Build history of the part. All positions in model axes, mm. Face numbers are marked on the shaded views. A direction names the side the tool comes from. Coordinates: 2 decimals unless noted, no trailing zeros. Loops run counter-clockwise (first coordinate to the right, second up) from the corner with the lowest first, then second, coordinate; pieces in that order, holes last. Notation, with made-up numbers: (7.5, -9.75) - (46.5, -9.75) arc R32 cw to (46.5, 21.25) - close; hole circle Ø8 at (34, -18.5). An arc over 180 degrees is marked (long way). One line per item, written item: value.
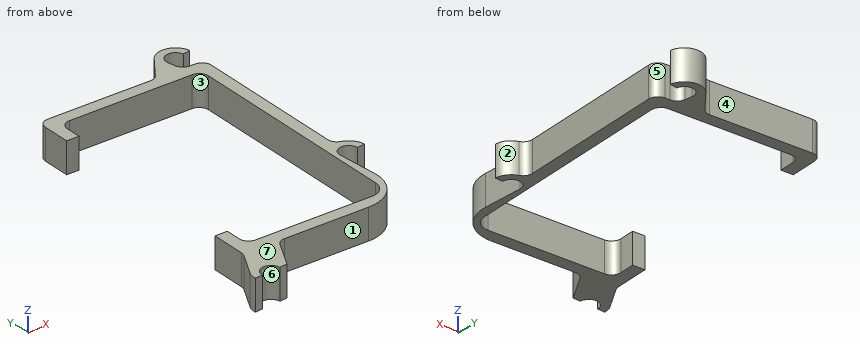
Autodesk Inventor part; units mm, degrees
ref_plane "YZ Plane" through (0, 0, 0) normal (1, 0, 0) x (0, 1, 0)
ref_plane "XZ Plane" through (0, 0, 0) normal (0, 1, 0) x (-1, 0, 0)
ref_plane "XY Plane" through (0, 0, 0) normal (0, 0, 1) x (1, 0, 0)
sketch "Sketch1" plane through (0, 0, 0) normal (0, 0, 1) x (1, 0, 0)
  arc A0 (1.905, 0) -> (-1.905, 0) centre (0, 0) ccw
  arc A1 (38.2001, 20.955) -> (34.3901, 20.9476) centre (36.2951, 20.955) ccw
  arc A2 (38.1877, 63.0819) -> (34.4025, 62.6481) centre (36.2951, 62.865) ccw
  line L0 (36.2951, 62.865) -> (36.2951, 20.955) construction
  line L1 (36.2951, 20.955) -> (0, 0) construction
  line L2 (32.146, 7.0452) -> (36.5038, 56.8549)
  line L3 (36.5038, 56.8549) -> (7.6142, 59.3825)
  line L4 (3.2564, 9.5727) -> (32.146, 7.0452)
  line L5 (0, 0) -> (62.4148, 0) construction
  line L6 (39.2555, 59.1639) -> (36.2181, 24.4467)
  line L7 (34.455, 4.2935) -> (7.7392, 6.6308)
  line L8 (7.1714, 54.3218) -> (4.6411, 54.5432)
  line L9 (3.6991, 14.6334) -> (1.1688, 14.8548)
  line L10 (38.2001, 20.955) -> (39.7876, 20.955)
  line L11 (-1.905, 0) -> (-3.4925, 0)
  line L12 (1.905, 0) -> (3.4925, 0)
  line L13 (0.5047, 7.2638) -> (1.1688, 14.8548)
  line L14 (4.6411, 54.5432) -> (5.3052, 62.1342)
  line L15 (7.6142, 59.3825) -> (7.1714, 54.3218)
  line L16 (3.6991, 14.6334) -> (3.2564, 9.5727)
  line L17 (0.5047, 7.2638) -> (-2.941, 1.8836)
  line L18 (3.4925, 0) -> (7.7392, 6.6308)
  line L19 (34.3901, 20.9476) -> (34.455, 4.2935)
  arc A3 (39.7876, 20.955) -> (36.2181, 24.4467) centre (36.2951, 20.955) ccw
  line L20 (33.6354, 65.1357) -> (29.2821, 60.0365)
  line L21 (38.1877, 63.0819) -> (39.7696, 63.2631)
  line L22 (34.4025, 62.6481) -> (34.7567, 59.5575)
  arc A4 (39.7696, 63.2631) -> (33.6354, 65.1357) centre (36.2951, 62.865) ccw
  arc A5 (-2.941, 1.8836) -> (-3.4925, 0) centre (0, 0) ccw
  line L23 (5.3052, 62.1342) -> (29.2821, 60.0365)
  line L24 (34.7567, 59.5575) -> (39.2555, 59.1639)
  dimension "d0" = 3.81
  dimension "d1" = 41.91
  dimension "d2" = 120
  dimension "d4" = 29
  dimension "d5" = 50
  dimension "d6" = 5.969
  dimension "d7" = 2.921
  dimension "d8" = 85
  dimension "d10" = 5.08
  dimension "d11" = 5.08
  dimension "d13" = 2.54
extrude "Extrusion1" add sketch "Sketch1" along normal blind 6.35
fillet "Fillet2" radius 3.175 1 edges at (32.146, 7.0452, 3.175)
fillet "Fillet1" radius 7.62 1 edges at (34.455, 4.2935, 3.175)
fillet "Fillet3" radius 1.905 10 edges at (3.2564, 9.5727, 3.175) (7.6142, 59.3825, 3.175) (36.5038, 56.8549, 3.175) (34.7567, 59.5575, 3.175) (29.2821, 60.0365, 3.175) (39.2555, 59.1639, 3.175) (36.2181, 24.4467, 3.175) (7.7392, 6.6308, 3.175) (0.5047, 7.2638, 3.175) (5.3052, 62.1342, 3.175)
equation "\"d13\" = d9"
properties part number "DriveBatteryHolder" material "ABS Plastic"
Item 1: Tool access for the marked faces 1, 2 and 3: list every direction of +Z, -Z, +X, -X, +Y, -Y with a clear straight run to the whole face (end or side of a thin tool).
Check result:
face 1: +Z, -Z, -Y
face 2: +Z, -Z, +X
face 3: +Z, -Z
Item 2: Pull direction Y, two halves, no side cores. Call the marked faces 4, 5, 6 and 7: released by +Y, released by -Y, zero draft, split by the parting line, or undercut.
Check result:
face 4: released by +Y
face 5: undercut
face 6: released by -Y
face 7: zero draft
Item 3: Cut at A-A, the plane y = 8.5. Write the cut outline in (x, z).
Check result:
outline: (0.61, 0) - (15.52, 0) - (15.52, 6.35) - (0.61, 6.35) - close; (31.74, 0) - (33.22, 0) - (33.22, 6.35) - (31.74, 6.35) - close
Item 4: Cut at C-C, the plane y = 53.5. Write the cut outline in (x, z).
Check result:
outline: (36.21, 0) - (38.76, 0) - (38.76, 6.35) - (36.21, 6.35) - close
Item 5: Drop flat-ended pins along their axis: P1, Ø2, axis at y = 33, z = 4.5, coming from the -X side; P2, Ø1.5, axis at y = 54, z = 5.5, coming from the -X side; P3, Ø1.3, axis at x = 39, z = 2, coming from the -Y side (3 decimals). Give the stop position or say it passes through.
Check result:
P1: stops at x = 34.33
P2: stops at x = 4.64
P3: stops at y = 20.955
Item 6: Probe probe 1 along Y at (x, z) = (15.5, 5.75); probe 2 along Y at (x, z) = (30, 3.5); probe 3 along Y at (x, z) = (4, 5.5). List the from-to ranges inside material, lowest first. Write a range as from..to.
Check result:
probe 1: y = 5.95..8.5, 58.69..61.24
probe 2: y = 5.7..7.4, 57.42..60.88
probe 3: y = 0.79..9.93
Item 7: Cut at B-B, the plane x = 13. Write the cut outline in (y, z).
Check result:
outline: (6.17, 0) - (8.72, 0) - (8.72, 6.35) - (6.17, 6.35) - close; (58.91, 0) - (61.46, 0) - (61.46, 6.35) - (58.91, 6.35) - close
